Verification items for the finished model (mm, model axes). A direction names the side the tool comes from. Give positions to 0.01 mm unless a question says otherwise; leave off trailing zeros. Loops run counter-clockwise (first coordinate to the right, second up) from the corner with the lowest first, then second, coordinate; pieces in that order, holes last. Notation, with made-up numbers: (-19, 40.5) - (15, 40.5) arc R10 ccw to (15, 49.5) - close; hole circle Ø8 at (56.5, 42.25). An arc over 180 degrees is marked (long way). Answer in a Markdown table with one row per item.
```python
from build123d import *

# Parameters (mm, degrees)
F0_W     = 50.8
F0_H     = 50.8
F1_DEPTH = 50.8
F2_W     = 26.1030352294
F2_H     = 25.92160739
F3_DEPTH = 50.8
F4_DEPTH = 25.4


with BuildPart() as f1:
    # F0 (on Front) → F1 (new body)
    with BuildSketch(Plane.XZ):
        with Locations((-25.4, 25.4)):
            Rectangle(F0_W, F0_H)
    extrude(amount=F1_DEPTH)

    # F2 (on face) → F3 (join)
    with BuildSketch(Plane.XZ.offset(50.8)):
        with Locations((-37.7484823853, 12.960803695)):
            Rectangle(F2_W, F2_H)
    extrude(amount=F3_DEPTH)

    # F4 (cut): a face of the model
    f4_faces = [f1.faces().sort_by_distance(p)[0] for p in [
        (-37.7484823853, -101.6, 12.960803695),
    ]]
    extrude(f4_faces, amount=-F4_DEPTH, mode=Mode.SUBTRACT)


solid = f1.part
```
Q1. Sectioned sample at D-D (x = -16.5). Record the cut outline in (y, z).
Completed:
| item | result |
|---|---|
| outline | (-50.8, 0) - (0, 0) - (0, 50.8) - (-50.8, 50.8) - close |
Q2. Thickness scan on line 1 (Y direction, x = -3.5, z = 21.5); line 2 (Z direction, x = -32.5, y = -52); line 3 (X direction, y = -55, z = 7). Record the ranges inside material, lowest first.
Completed:
| item | result |
|---|---|
| line 1 | -50.8 to 0 |
| line 2 | 0 to 25.92 |
| line 3 | -50.8 to -24.7 |
Q3. Sectioned sample at B-B (x = -29). Record the cut outline in (y, z).
Completed:
| item | result |
|---|---|
| outline | (-76.2, 0) - (0, 0) - (0, 50.8) - (-50.8, 50.8) - (-50.8, 25.92) - (-76.2, 25.92) - close |
Q4. Sectioned sample at A-A (z = 31.5). Record the cut outline in (x, y), and give its area (3 significant figures).
Completed:
| item | result |
|---|---|
| outline | (-50.8, -50.8) - (0, -50.8) - (0, 0) - (-50.8, 0) - close |
| area | 2,580 mm^2 |
Q5. Sectioned sample at C-C (z = 25). Record the cut outline in (x, y), and give its area (3 significant figures).
Completed:
| item | result |
|---|---|
| outline | (-50.8, -76.2) - (-24.7, -76.2) - (-24.7, -50.8) - (0, -50.8) - (0, 0) - (-50.8, 0) - close |
| area | 3,240 mm^2 |
Q6. Go/stop test with flat-tipped pins: P1, Ø12.5, axis at y = -60.5, z = 8, coming from the +X side; P2, Ø2, axis at y = -9.5, z = 39, coming from the +X side; P3, Ø8, axis at x = -7, z = 9.5, coming from the -Y side. Record where each tip stops, or that it passes through.
Completed:
| item | result |
|---|---|
| P1 | x = -24.7 |
| P2 | x = 0 |
| P3 | y = -50.8 |
Q7. Tool access check on faces 1 (the face through (-24.697, -63, 13)), 2 (the face through (0, -25, 25)), 3 (the face through (-38, -63, 25.922)). Record the directions out of +Z, -Z, +X, -X, +Y, -Y that give a thin tool (end or side, any length) a straight path to the whole face; none if there is none.
Completed:
| item | result |
|---|---|
| face 1 | +Z, -Z, +X, -Y |
| face 2 | +Z, -Z, +X, +Y, -Y |
| face 3 | +Z, +X, -X, -Y |
